Geometry: final body of the model. Coordinates: model frame, mm. Face numbers are marked on the shaded views. A direction names the side the tool comes from. Give positions to 0.01 mm unless a question says otherwise; leave off trailing zeros. Loops run counter-clockwise (first coordinate to the right, second up) from the corner with the lowest first, then second, coordinate; pieces in that order, holes last.
1. Access query for the marked faces 1 and 2. Directions: +Z, -Z, +X, -X, +Y, -Y. A direction counts if a zero-diameter tool reaches every point of the face in a straight line with its end or side. Return the directions, or none.
2. First-contact query: P1, Ø1.7, axis at x = -15.24, y = -3.21, coming from the -Z side; P2, Ø5, axis at y = -36.5, z = -0.5, coming from the -X side. Flat tips, straight axial feed; report the tip coordinate or a pass-through.
3. Section B-B, the plane x = 5. Output: boundary loops of the cut face in (y, z).
4. Section D-D, the plane z = 9.5. Output: boundary loops of the cut face in (x, y), then the cut area to 3 significant figures.
5. Draft query along Y for the marked faces 3, 4 and 5. Return one class per face: +Y half, -Y half, draft (parallel to the pull), parting line (faces both ways), or undercut.
6. Section C-C, the plane y = 38.1. Output: boundary loops of the cut face in (x, z), then the cut area to 3 significant figures.
7. Material intervals for line 1 along Z through (x, y) = (16.5, 5.5); line 2 along Y through (x, z) = (17, 2.75); line 3 along Y through (x, z) = (-15.24, -9.5), sorted ascending.
8. Section A-A, the plane z = 0. Output: boundary loops of the cut face in (x, y).
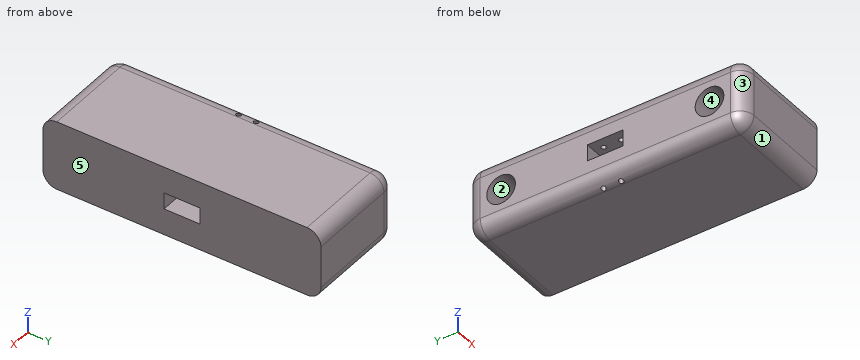
from build123d import *

# Parameters (mm, degrees)
F0_W     = 38.1
F0_H     = 101.6
F1_DEPTH = 12.7
F2_R     = 5.23875
F3_DEPTH = 25.4
F4_R     = 5.08
F5_W     = 13.081
F5_H     = 6.0452
F6_DEPTH = 38.1
F8_DEPTH = 25.401


with BuildPart() as f1:
    # F0 (on Top) → F1 (new body, symmetric)
    with BuildSketch(Plane.XY):
        Rectangle(F0_W, F0_H)
    extrude(amount=F1_DEPTH, both=True)

    # F2 (on face) → F3 (cut)
    with BuildSketch(Plane(origin=(-19.05, 0, 0), x_dir=(0, -1, 0), z_dir=(-1, 0, 0))):
        with Locations((38.1, 0)):
            Circle(F2_R)
        with Locations((-38.1, 0)):
            Circle(F2_R)
    extrude(amount=-F3_DEPTH, mode=Mode.SUBTRACT)

    # F4
    f4_edges = [f1.edges().sort_by_distance(p)[0] for p in [
        (0, 50.8, 12.7),
        (-19.05, 0, 12.7),
        (-19.05, 50.8, 0),
        (-19.05, -50.8, 0),
        (-19.05, 0, -12.7),
        (0, 50.8, -12.7),
        (0, -50.8, -12.7),
        (0, -50.8, 12.7),
    ]]
    fillet(f4_edges, radius=F4_R)

    # F5 (on face) → F6 (cut, through all)
    with BuildSketch(Plane(origin=(-19.05, 0, 0), x_dir=(0, -1, 0), z_dir=(-1, 0, 0))):
        Rectangle(F5_W, F5_H)
    extrude(amount=-F6_DEPTH, mode=Mode.SUBTRACT)

    # F7 (on face) → F8 (cut, through all)
    with BuildSketch(Plane.XY.offset(12.7)):
        with BuildLine():
            ThreePointArc((-14.31925, -3.20675), (-14.588931, -2.555681), (-15.24, -2.286))
            ThreePointArc((-15.24, -2.286), (-15.891069, -3.857819), (-14.31925, -3.20675))
        make_face()
        with BuildLine():
            ThreePointArc((-14.31925, 3.20675), (-15.891069, 3.857819), (-15.24, 2.286))
            ThreePointArc((-15.24, 2.286), (-14.588931, 2.555681), (-14.31925, 3.20675))
        make_face()
    extrude(amount=-F8_DEPTH, mode=Mode.SUBTRACT)


solid = f1.part
Answers below:
1. face 1: -Z, +X, -X, -Y
1. face 2: -X
2. P1: passes through
2. P2: stops at x = 6.35
3. outline: (-50.8, -7.62) arc R5.08 ccw to (-45.72, -12.7) - (45.72, -12.7) arc R5.08 ccw to (50.8, -7.62) - (50.8, 7.62) arc R5.08 ccw to (45.72, 12.7) - (-45.72, 12.7) arc R5.08 ccw to (-50.8, 7.62) - close; hole circle Ø10.48 at (-38.1, 0); hole (-6.54, -3.02) - (6.54, -3.02) - (6.54, 3.02) - (-6.54, 3.02) - close; hole circle Ø10.48 at (38.1, 0)
4. outline: (-18.69, -45.72) arc R4.72 ccw to (-13.97, -50.44) - (19.05, -50.44) - (19.05, 50.44) - (-13.97, 50.44) arc R4.72 ccw to (-18.69, 45.72) - close; hole (-15.24, -2.29) arc R0.92 ccw (long way) to (-14.32, -3.21) arc R0.92 ccw to start; hole (-15.24, 2.29) arc R0.92 ccw to (-14.32, 3.21) arc R0.92 ccw (long way) to start
4. area: 3,790 mm2
5. face 3: -Y half
5. face 4: undercut
5. face 5: draft
6. outline: (-19.05, -7.62) arc R5.08 ccw to (-13.97, -12.7) - (19.05, -12.7) - (19.05, 12.7) - (-13.97, 12.7) arc R5.08 ccw to (-19.05, 7.62) - (-19.05, 5.24) - (6.35, 5.24) - (6.35, -5.24) - (-19.05, -5.24) - close
6. area: 691 mm2
7. line 1: z = -12.7 to -3.02, 3.02 to 12.7
7. line 2: y = -50.8 to -6.54, 6.54 to 50.8
7. line 3: y = -50.27 to -4.13, -2.29 to 2.29, 4.13 to 50.27
8. outline: (-19.05, -45.72) arc R5.08 ccw to (-13.97, -50.8) - (19.05, -50.8) - (19.05, -6.54) - (-19.05, -6.54) - (-19.05, -32.86) - (6.35, -32.86) - (6.35, -43.34) - (-19.05, -43.34) - close; (-19.05, 6.54) - (19.05, 6.54) - (19.05, 50.8) - (-13.97, 50.8) arc R5.08 ccw to (-19.05, 45.72) - (-19.05, 43.34) - (6.35, 43.34) - (6.35, 32.86) - (-19.05, 32.86) - close
